from build123d import *

# Parameters (mm, degrees)
ESQUISSE1_W          = 370
ESQUISSE1_H          = 25
ESQUISSE1_W_2        = 340
ESQUISSE1_H_2        = 10
BOSS_EXTRU_1_DEPTH   = 3
D_GAGEMENT_M51_D     = 5.8
D_GAGEMENT_M51_DEPTH = 4


with BuildPart() as part:
    # Esquisse1 → Boss.-Extru.1 (new body)
    with BuildSketch(Plane(origin=(0, 0, 0), x_dir=(1, 0, 0), z_dir=(0, 1, 0))):
        Rectangle(ESQUISSE1_W, ESQUISSE1_H)
        Rectangle(ESQUISSE1_W_2, ESQUISSE1_H_2, mode=Mode.SUBTRACT)
    extrude(amount=BOSS_EXTRU_1_DEPTH)

    # Dégagement M51
    with Locations(Plane(origin=(0, 3, 0), x_dir=(1, 0, 0), z_dir=(0, 1, 0))):
        with Locations((-180, 7.5), (-180, -7.5), (180, -7.5), (180, 7.5)):
            Hole(D_GAGEMENT_M51_D / 2, depth=D_GAGEMENT_M51_DEPTH)


solid = part.part
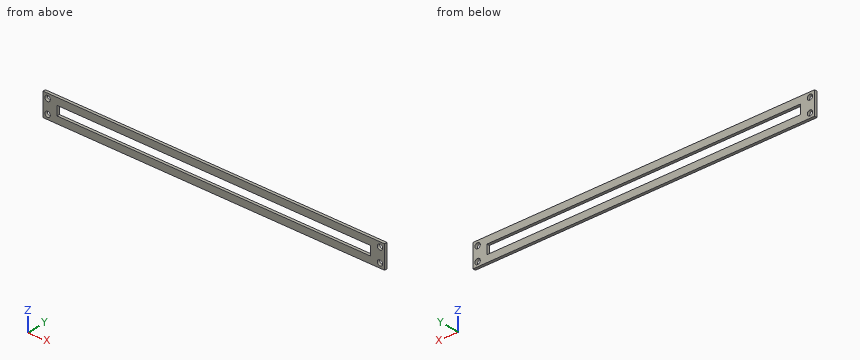
The listing builds one solid part. Answer for the finished solid, in the listing's coordinates (mm). Round coordinates to 2 decimals unless told otherwise and drop trailing zeros. Order: outer loops, then holes, each group sorted by start corner. A loop starts at its lowest first (then second) coordinate and runs counter-clockwise, first axis right, second up. Notation, with made-up numbers: M 41,26 L 64,26 A20 cw 64,55 Z; hole C 78,-30.75 d6. An arc over 180 degrees is marked long. Answer in a Markdown table with one row per item. Add a question column.
1) The part is cut by section C-C on y = 0.85. Determine the outline of the cut face in (x, z), plus the area to 3 significant figures.
2) The part is cut by section A-A on z = -0.5. Determine the outline of the cut face in (x, y), plus the area to 3 significant figures.
3) The part is cut by section B-B on x = 130.5. Determine the outline of the cut face in (y, z).
4) Consider line 1 along X through (y, z) = (1.4, 8); line 2 along Z through (x, y) = (180, 0.7); line 3 along X through (y, z) = (0.8, -3.5). Determine where each line is inside the solid, lowest interval first. Write a range as from..to.
Findings below:
| question | item | result |
|---|---|---|
| 1 | outline | M -185,-12.5 L 185,-12.5 L 185,12.5 L -185,12.5 Z; hole C -180,-7.5 d5.8; hole C -180,7.5 d5.8; hole M -170,-5 L 170,-5 L 170,5 L -170,5 Z; hole C 180,-7.5 d5.8; hole C 180,7.5 d5.8 |
| 1 | area | 5,740 mm² |
| 2 | outline | M -185,0 L -170,0 L -170,3 L -185,3 Z; M 170,0 L 185,0 L 185,3 L 170,3 Z |
| 2 | area | 90.0 mm² |
| 3 | outline | M 0,-12.5 L 3,-12.5 L 3,-5 L 0,-5 Z; M 0,5 L 3,5 L 3,12.5 L 0,12.5 Z |
| 4 | line 1 | x = -185..-182.86, -177.14..177.14, 182.86..185 |
| 4 | line 2 | z = -12.5..-10.4, -4.6..4.6, 10.4..12.5 |
| 4 | line 3 | x = -185..-170, 170..185 |
